Read the model definition and answer for the solid it produces. Units are mm, in the model's axes. Face numbers are marked on the shaded views. Give positions to 0.01 mm unless a question says otherwise; leave off trailing zeros. Order: outer loops, then holes, each group sorted by start corner. A loop starts at its lowest first (then second) coordinate and runs counter-clockwise, first axis right, second up.
Item 1: A cutting plane is placed at C-C (y = 37). Write down the section's boundary in (x, z).
Item 2: A cutting plane is placed at A-A (y = 109.5). Write down the section's boundary in (x, z) (1 decimal).
Item 3: A cutting plane is placed at D-D (z = 0). Write down the section's boundary in (x, y), plus the area to 3 significant figures.
Item 4: Find the intervals of material crossed by line 1 along Z through (x, y) = (-1.5, 79.5) (1 decimal); line 2 along Z through (x, y) = (-3.5, 26); line 3 along Y through (x, z) = (-9, 15), in increasing order.
Item 5: The mould has two halves that part along Z. Classify the marked faces 1, 2, 3 and 4: +Z half, -Z half, draft (parallel to the pull), parting line (faces both ways), or undercut.
Item 6: Given pin 1 Ø5 at (x, y) = (18.5, 31.5) entering from +Z; pin 2 Ø2 at (x, z) = (14, -3.5) entering from +Y; pin 3 Ø8 at (x, z) = (3.5, -3) entering from +Y, each flat-ended and moving along its own axis, determine where each tip first touches the part or whether it passes through.
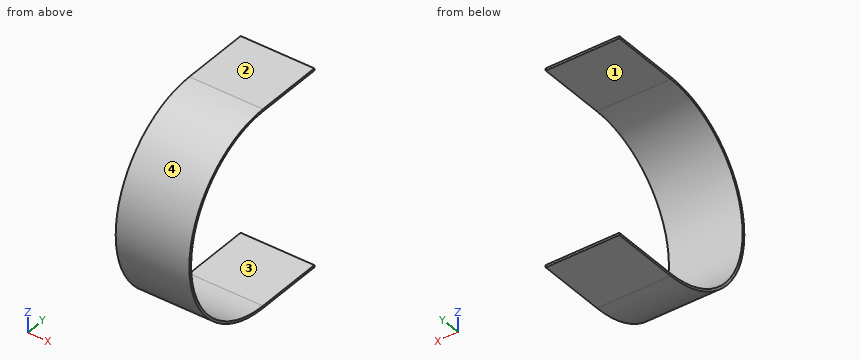
Autodesk Inventor part; units mm, degrees
ref_plane "YZ Plane" through (0, 0, 0) normal (1, 0, 0) x (0, 1, 0)
ref_plane "XZ Plane" through (0, 0, 0) normal (0, 1, 0) x (-1, 0, 0)
ref_plane "XY Plane" through (0, 0, 0) normal (0, 0, 1) x (1, 0, 0)
sketch "Sketch1" plane through (0, 0, 0) normal (0, 1, 0) x (-1, 0, 0)
  line L0 (25.4, -152.4) -> (-25.4, -152.4)
  line L1 (-25.4, -152.4) -> (-25.4, 152.4)
  line L2 (-25.4, 152.4) -> (25.4, 152.4)
  line L3 (25.4, 152.4) -> (25.4, -152.4)
  line L4 (25.4, -152.4) -> (-25.4, 152.4) construction
  line L5 (-25.4, -152.4) -> (25.4, 152.4) construction
  point P0 (0, 0)
  dimension "d0" = 50.8
  dimension "d1" = 304.8
extrude "Extrusion1" add sketch "Sketch1" along normal blind 1.5875
sketch "Sketch2" plane through (0, 1.5875, 0) normal (0, 1, 0) x (1, 0, 0)
  line L0 (25.4, -152.4) -> (25.4, 152.4)
  line L1 (-54.3689, 0) -> (59.0967, 0)
  line L2 (-25.4, -152.4) -> (25.4, 152.4) construction
  line L3 (-25.4, 152.4) -> (25.4, -152.4) construction
  point P0 (0, 0)
  point P1 (0, 0)
bend part "Bend Part1" radius 66.675 angle 180 line through (-54.3689, 1.5875, 0) along (1, 0, 0) centre toward (0, 1, 0) moving side (0, 0, -1) both sides yes
properties part number "side" material "Polycarbonate, Clear"
Response values:
1. outline: (-25.4, -60.68) - (25.4, -60.68) - (25.4, -58.89) - (-25.4, -58.89) - close; (-25.4, 58.89) - (25.4, 58.89) - (25.4, 60.68) - (-25.4, 60.68) - close
2. outline: (-25.4, -68.3) - (25.4, -68.3) - (25.4, -66.7) - (-25.4, -66.7) - close; (-25.4, 66.7) - (25.4, 66.7) - (25.4, 68.3) - (-25.4, 68.3) - close
3. outline: (-25.4, 0) - (25.4, 0) - (25.4, 1.59) - (-25.4, 1.59) - close
3. area: 80.6 mm2
4. line 1: z = -68.3 to -66.7, 66.7 to 68.3
4. line 2: z = -53.61 to -51.57, 51.57 to 53.61
4. line 3: y = 1.67 to 3.3
5. face 1: undercut
5. face 2: +Z half
5. face 3: undercut
5. face 4: parting line
6. pin 1: stops at z = 59.04
6. pin 2: stops at y = 1.74
6. pin 3: stops at y = 1.96
